Part model, mm, in its own coordinate system. A direction names the side the tool comes from. Round coordinates to 2 decimals unless told otherwise and drop trailing zeros. Write each loop counter-clockwise with the first axis right and the second up, starting at its lowest first coordinate (ties: lowest second). Pieces come first, ordered by that corner, then holes. Notation, with made-up numbers: M 73.5,16 L 107.5,16 A23 ccw 107.5,53 Z; hole C 45,74 d8. An arc over 180 degrees is marked long. Use one line per item in the form item = value. Start each with the question number.
Item 1: Cut at A-A, the plane x = 0. Give the cut face in (y, z) (1 decimal).
Item 2: Cut at C-C, the plane z = 2.6. Give the cut face in (x, y) (1 decimal).
Item 3: Cut at D-D, the plane x = 8.5. Give the cut face in (y, z) (3 decimals).
Item 4: Which spindle directions (+Z, -Z, +X, -X, +Y, -Y) get a long thin tool onto all of the face, cutting with end or side? Do faces 1 (the face through (-14.415, -11.212, 1.61)), 2 (the face through (-16.066, 14, 2)), 3 (the face through (16.066, 14, 2)). Say none if no direction does.
Item 5: Mould opens along Y. For faces 4 (the face through (-18.52, -8.76, 1.61)), 5 (the face through (14.415, -11.212, 1.61)), 6 (the face through (10.6, 3.34, 1.57)), 7 (the face through (-19.24, 0, 2)) say: +Y half, -Y half, draft (parallel to the pull), parting line (faces both ways), or undercut.
Item 6: Probe L1, parallel to Y at x = 0, z = 1.15 (1 decimal); L2, parallel to Y at x = 2, z = 2.2 (3 decimals); L3, parallel to X at y = 0.5, z = 1.3. List the from-to ranges inside material, lowest first.
Item 7: Flat gauge pins, fed straight in: pin 1 Ø1.5 at (y, z) = (13.5, 1.5) entering from +X; pin 2 Ø1.5 at (y, z) = (13.5, 1.5) entering from -X; pin 3 Ø1.5 at (x, y) = (-10, 1) entering from -Z. Where does each tip first touch, or does it go through?
Item 8: Cut at B-B, the plane y = -1. Give the cut face in (x, z) (1 decimal).
from build123d import *

# Parameters (mm, degrees)
SKETCH1_R           = 11.1125
BOSS_EXTRUDE1_DEPTH = 3.175
BOSS_EXTRUDE3_DEPTH = 3.175
SKETCH4_R           = 2.5527
CUT_EXTRUDE2_DEPTH  = 4.175
FILLET1_R           = 2.54
CUT_EXTRUDE1_DEPTH  = 4.175


with BuildPart() as part:
    # Sketch1 → Boss-Extrude1 (new body)
    with BuildSketch(Plane.XY):
        Polygon((-19.2405, -9.525), (-19.2405, 9.525), (-16.0655, 9.525), (-16.0655, 15.875), (16.0655, 15.875), (16.0655, 9.525), (19.2405, 9.525), (19.2405, -9.525), (16.0655, -9.525), (16.0655, -15.875), (-16.0655, -15.875), (-16.0655, -9.525), align=None)
        Circle(SKETCH1_R, mode=Mode.SUBTRACT)
    extrude(amount=BOSS_EXTRUDE1_DEPTH)

    # Sketch3 → Boss-Extrude3 (add)
    with BuildSketch(Plane.XY.offset(3.175)):
        with BuildLine():
            Line((-16.0655, 15.875), (16.0655, 15.875))
            ThreePointArc((16.0655, 15.875), (0, 22.529547986), (-16.0655, 15.875))
        make_face()
    extrude(amount=-BOSS_EXTRUDE3_DEPTH)

    # Sketch4 → Cut-Extrude2 (cut, through all)
    with BuildSketch(Plane(origin=(0, 0, 0), x_dir=(-1, 0, 0), z_dir=(0, 0, -1))):
        with Locations((0, 15.875)):
            Circle(SKETCH4_R)
    extrude(amount=-CUT_EXTRUDE2_DEPTH, mode=Mode.SUBTRACT)

    # Fillet1
    fillet1_edges = [part.edges().sort_by_distance(p)[0] for p in [
        (19.2405, 9.525, 1.5875),
        (19.2405, -9.525, 1.5875),
        (16.0655, -15.875, 1.5875),
        (-16.0655, -15.875, 1.5875),
        (-19.2405, -9.525, 1.5875),
        (-19.2405, 9.525, 1.5875),
    ]]
    fillet(fillet1_edges, radius=FILLET1_R)

    # Sketch2 → Cut-Extrude1 (cut, through all)
    with BuildSketch(Plane.XY.offset(3.175)):
        with BuildLine():
            Line((-16.0655, -9.525), (-16.0655, -12.827))
            ThreePointArc((-16.0655, -12.827), (-14.4145, -11.176), (-16.0655, -9.525))
        make_face()
        with BuildLine():
            Line((16.0655, -9.525), (16.0655, -12.827))
            ThreePointArc((16.0655, -12.827), (14.4145, -11.176), (16.0655, -9.525))
        make_face()
        with BuildLine():
            Line((-16.0655, 9.525), (-16.0655, 12.827))
            ThreePointArc((-16.0655, 12.827), (-14.4145, 11.176), (-16.0655, 9.525))
        make_face()
        with BuildLine():
            Line((16.0655, 9.525), (16.0655, 12.827))
            ThreePointArc((16.0655, 12.827), (14.4145, 11.176), (16.0655, 9.525))
        make_face()
    extrude(amount=-CUT_EXTRUDE1_DEPTH, mode=Mode.SUBTRACT)


solid = part.part
Model answer:
q1.outline = M -15.9,0 L -11.1,0 L -11.1,3.2 L -15.9,3.2 Z; M 11.1,0 L 13.3,0 L 13.3,3.2 L 11.1,3.2 Z; M 18.4,0 L 22.5,0 L 22.5,3.2 L 18.4,3.2 Z
q2.outline = M -19.2,-7 A2.5 ccw -16.7,-9.5 L -16.1,-9.5 A1.7 cw -16.1,-12.8 L -16.1,-13.3 A2.5 ccw -13.5,-15.9 L 13.5,-15.9 A2.5 ccw 16.1,-13.3 L 16.1,-12.8 A1.7 cw 16.1,-9.5 L 16.7,-9.5 A2.5 ccw 19.2,-7 L 19.2,7 A2.5 ccw 16.7,9.5 L 16.1,9.5 A1.7 cw 16.1,12.8 L 16.1,15.9 A22.7 ccw -16.1,15.9 L -16.1,12.8 A1.7 cw -16.1,9.5 L -16.7,9.5 A2.5 ccw -19.2,7 Z; hole C 0,0 d22.2; hole C 0,15.9 d5.1
q3.outline = M -15.875,0 L -7.158,0 L -7.158,3.175 L -15.875,3.175 Z; M 7.158,0 L 20.88,0 L 20.88,3.175 L 7.158,3.175 Z
q4.face_1 = +Z, -Z, -X
q4.face_2 = +Z, -Z, -X, +Y
q4.face_3 = +Z, -Z, +X, +Y
q5.face_4 = -Y half
q5.face_5 = undercut
q5.face_6 = undercut
q5.face_7 = draft
q6.L1 = -15.9 to -11.1, 11.1 to 13.3, 18.4 to 22.5
q6.L2 = -15.875 to -10.931, 10.931 to 14.289, 17.461 to 22.441
q6.L3 = -19.24 to -11.1, 11.1 to 19.24
q7.pin_1 = 16.07
q7.pin_2 = -16.07
q7.pin_3 = through
q8.outline = M -19.2,0 L -11.1,0 L -11.1,3.2 L -19.2,3.2 Z; M 11.1,0 L 19.2,0 L 19.2,3.2 L 11.1,3.2 Z
